CAD build for the part. Positions are in the model's coordinates, mm. Face numbers are marked on the shaded views. A direction names the side the tool comes from. Round coordinates to 2 decimals unless told otherwise and drop trailing zeros. Order: outer loops, then holes, each group sorted by start corner. A loop starts at its lowest first (then second) coordinate and runs counter-clockwise, first axis right, second up. Notation, with made-up numbers: M -25,2.25 L 14,2.25 A11 cw 14,7.25 Z; hole C -18.5,55 d7. An arc over 180 degrees is marked long. Put each result on its own line as item: value.
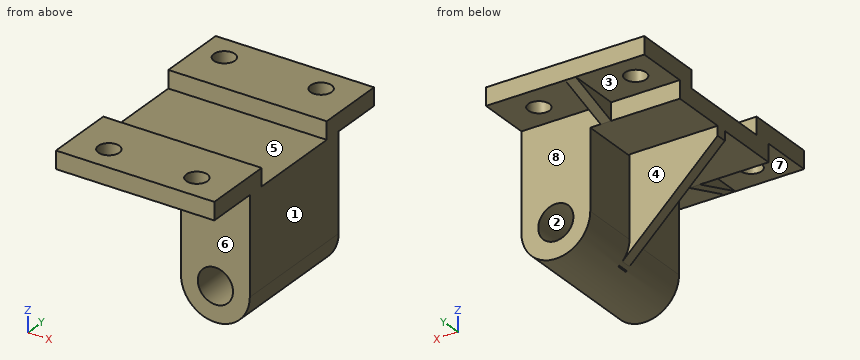
```python
from build123d import *

# Parameters (mm, degrees)
SKETCH4_W           = 90
SKETCH4_H           = 10
BOSS_EXTRUDE3_DEPTH = 135
BOSS_EXTRUDE4_DEPTH = 90
SKETCH6_W           = 10
SKETCH6_H           = 55
CUT_EXTRUDE3_DEPTH  = 130
BOSS_EXTRUDE5_DEPTH = 75
SKETCH8_R           = 10
CUT_EXTRUDE4_DEPTH  = 95
SKETCH11_R          = 6
CUT_EXTRUDE5_DEPTH  = 95
SKETCH12_R          = 6
CUT_EXTRUDE6_DEPTH  = 95
SKETCH13_W          = 6
SKETCH13_H          = 10
BOSS_EXTRUDE6_DEPTH = 30
CUT_EXTRUDE7_DEPTH  = 30
BOSS_EXTRUDE7_DEPTH = 3
CUT_EXTRUDE10_DEPTH = 18
SKETCH18_W          = 6
SKETCH18_H          = 10
BOSS_EXTRUDE8_DEPTH = 30
CUT_EXTRUDE11_DEPTH = 30
SKETCH20_W          = 50.090708896
SKETCH20_H          = 1.471886497
BOSS_EXTRUDE9_DEPTH = 6
SKETCH21_W          = 9.793244498
SKETCH21_H          = 5.326709205
CUT_EXTRUDE12_DEPTH = 6


with BuildPart() as part:
    # Sketch4 → Boss-Extrude3 (new body)
    with BuildSketch(Plane(origin=(0, 0, 0), x_dir=(1, 0, 0), z_dir=(0, 1, 0))):
        with Locations((45, 5)):
            Rectangle(SKETCH4_W, SKETCH4_H)
    extrude(amount=BOSS_EXTRUDE3_DEPTH)

    # Sketch5 → Boss-Extrude4 (add)
    with BuildSketch(Plane(origin=(0, 0, 0), x_dir=(0, 0, -1), z_dir=(1, 0, 0))):
        Polygon((0, 0), (0, 40), (10, 40), (10, 95), (0, 95), (0, 135), (10, 135), (10, 105), (20, 105), (20, 30), (10, 30), (10, 0), align=None)
    extrude(amount=BOSS_EXTRUDE4_DEPTH)

    # Sketch6 → Cut-Extrude3 (cut)
    with BuildSketch(Plane.ZY):
        with Locations((-5, 67.5)):
            Rectangle(SKETCH6_W, SKETCH6_H)
    extrude(amount=-CUT_EXTRUDE3_DEPTH, mode=Mode.SUBTRACT)

    # Sketch7 → Boss-Extrude5 (add)
    with BuildSketch(Plane.XZ.offset(-30)):
        with BuildLine():
            Line((90, -20), (90, -65))
            ThreePointArc((90, -65), (70.445832322, -84.554167678), (50.891664643, -65))
            Line((50.891664643, -65), (50.891664643, -20))
            Line((50.891664643, -20), (90, -20))
        make_face()
    extrude(amount=-BOSS_EXTRUDE5_DEPTH)

    # Sketch8 → Cut-Extrude4 (cut)
    with BuildSketch(Plane.XZ.offset(-30)):
        with Locations((70.445832322, -65)):
            Circle(SKETCH8_R)
    extrude(amount=-CUT_EXTRUDE4_DEPTH, mode=Mode.SUBTRACT)

    # Sketch11 → Cut-Extrude5 (cut)
    with BuildSketch(Plane(origin=(0, 0, -10), x_dir=(-1, 0, 0), z_dir=(0, 0, -1))):
        with Locations((-70, 15)):
            Circle(SKETCH11_R)
        with Locations((-20, 15)):
            Circle(SKETCH11_R)
    extrude(amount=-CUT_EXTRUDE5_DEPTH, mode=Mode.SUBTRACT)

    # Sketch12 → Cut-Extrude6 (cut)
    with BuildSketch(Plane(origin=(0, 0, -10), x_dir=(-1, 0, 0), z_dir=(0, 0, -1))):
        with Locations((-70, 120)):
            Circle(SKETCH12_R)
        with Locations((-15, 120)):
            Circle(SKETCH12_R)
    extrude(amount=-CUT_EXTRUDE6_DEPTH, mode=Mode.SUBTRACT)

    # Sketch13 → Boss-Extrude6 (add)
    with BuildSketch(Plane.XZ.offset(-30)):
        with Locations((42, -15)):
            Rectangle(SKETCH13_W, SKETCH13_H)
    extrude(amount=BOSS_EXTRUDE6_DEPTH)

    # Sketch14 → Cut-Extrude7 (cut)
    with BuildSketch(Plane.ZY.offset(-39)):
        Polygon((-20, 30), (-9.033737426, -2.819084872), (-23.067852081, -4.027904728), (-23.067852081, 30), align=None)
    extrude(amount=-CUT_EXTRUDE7_DEPTH, mode=Mode.SUBTRACT)

    # Sketch16 → Boss-Extrude7 (add, symmetric)
    with BuildSketch(Plane(origin=(0, 70, 0), x_dir=(1, 0, 0), z_dir=(0, 1, 0))):
        with BuildLine():
            Line((50.090708896, 21.471886497), (50.090708896, 65.894352206))
            ThreePointArc((50.090708896, 65.894352206), (51.806699753, 73.025071947), (56.578931041, 78.594416359))
            Line((56.578931041, 78.594416359), (-4.085392515, 78.594416359))
            Line((-4.085392515, 78.594416359), (-4.085392515, 21.471886497))
            Line((-4.085392515, 21.471886497), (50.090708896, 21.471886497))
        make_face()
    extrude(amount=BOSS_EXTRUDE7_DEPTH, both=True)

    # Sketch17 → Cut-Extrude10 (cut, symmetric)
    with BuildSketch(Plane.XZ.offset(-67)):
        Polygon((55.920281495, -78.090983416), (-4.085392515, -21.471886497), (-4.085392515, -120.610546036), (55.920281495, -116.406239738), align=None)
    extrude(amount=CUT_EXTRUDE10_DEPTH, both=True, mode=Mode.SUBTRACT)

    # Sketch18 → Boss-Extrude8 (add)
    with BuildSketch(Plane(origin=(0, 105, 0), x_dir=(1, 0, 0), z_dir=(0, 1, 0))):
        with Locations((42, 15)):
            Rectangle(SKETCH18_W, SKETCH18_H)
    extrude(amount=BOSS_EXTRUDE8_DEPTH)

    # Sketch19 → Cut-Extrude11 (cut)
    with BuildSketch(Plane.ZY.offset(-39)):
        Polygon((-20, 105), (-10, 135), (-32.228945025, 136.35277526), (-34.026284176, 106.818709731), align=None)
    extrude(amount=-CUT_EXTRUDE11_DEPTH, mode=Mode.SUBTRACT)

    # Sketch20 → Boss-Extrude9 (add)
    with BuildSketch(Plane.XZ.offset(-67)):
        with Locations((25.045354448, -20.735943248)):
            Rectangle(SKETCH20_W, SKETCH20_H)
    extrude(amount=-BOSS_EXTRUDE9_DEPTH)

    # Sketch21 → Cut-Extrude12 (cut)
    with BuildSketch(Plane.XZ.offset(-67)):
        with Locations((-4.896622249, -22.663354603)):
            Rectangle(SKETCH21_W, SKETCH21_H)
    extrude(amount=-CUT_EXTRUDE12_DEPTH, mode=Mode.SUBTRACT)


solid = part.part
```
Item 1: Probe line 1 along Y through (x, z) = (70, -8); line 2 along Y through (x, z) = (84, -56.5); line 3 along Z through (x, y) = (27.5, 89). List the from-to ranges inside material, lowest first. Write a range as [from, to].
Answers below:
line 1: [0, 9], [21, 40], [95, 114], [126, 135]
line 2: [30, 105]
line 3: [-20, -10]
Item 2: Band-saw the part on B-B on z = -51. Give the cut face in (x, y), and give its area (3 significant figures).
Answers below:
outline: M 27.21,67 L 50.09,67 L 50.09,73 L 27.21,73 Z; M 50.89,30 L 90,30 L 90,105 L 50.89,105 Z
area: 3,070 mm²
Item 3: Tool access for the marked faces 4, 5, 6, 7 and 8: list every direction of +Z, -Z, +X, -X, +Y, -Y with a clear straight run to the whole face (end or side of a thin tool).
Answers below:
face 4: -Z, -X, +Y
face 5: +Z, +X, -X
face 6: -Z, +X, -Y
face 7: -Z, -X, -Y
face 8: -Z, +X, +Y
Item 4: Mould opens along Z. For the marked faces 1, 2 and 3 say: pulls with the +Z half, pulls with the -Z half, needs draft (parallel to the pull), parting line crosses it, or undercut.
Answers below:
face 1: needs draft
face 2: undercut
face 3: pulls with the -Z half
Item 5: Band-saw the part on A-A on y = 120. Give the cut face in (x, z), and give its area (3 significant figures).
Answers below:
outline: M 0,-10 L 9,-10 L 9,0 L 0,0 Z; M 21,-10 L 39,-10 L 39,-15 L 45,-15 L 45,-10 L 64,-10 L 64,0 L 21,0 Z; M 76,-10 L 90,-10 L 90,0 L 76,0 Z
area: 690 mm²
Item 6: Pin check, flat tips, straight feed: P1, Ø3, axis at y = 11.5, z = -15, coming from the +X side; P2, Ø12, axis at x = 39, z = -10, coming from the -Y side; P3, Ø2, axis at x = 34, z = -41.5, coming from the +Y side; P4, Ø15, axis at x = 71, y = 122, coming from the -Z side. Stop position of each tip, or through.
Answers below:
P1: x = 45
P2: y = 0
P3: y = 73
P4: z = -10
Item 7: Band-saw the part on D-D on y = 11.5. Give the cut face in (x, z).
Answers below:
outline: M 0,-10 L 15.13,-10 L 15.13,0 L 0,0 Z; M 24.87,-10 L 39,-10 L 39,-13.82 L 45,-13.82 L 45,-10 L 65.13,-10 L 65.13,0 L 24.87,0 Z; M 74.87,-10 L 90,-10 L 90,0 L 74.87,0 Z
Item 8: Band-saw the part on C-C on z = -73.5. Give the cut face in (x, y).
Answers below:
outline: M 51.05,67 L 52.06,67 L 52.06,73 L 51.05,73 Z; M 52.84,30 L 65.18,30 L 65.18,105 L 52.84,105 Z; M 75.71,30 L 88.06,30 L 88.06,105 L 75.71,105 Z
